Can you work these out from the model? Positions are in its coordinate system, mm. A direction names the side the tool comes from. Coordinates: 2 decimals unless noted, no trailing zeros. Order: outer loops, then holes, each group sorted by start corner. A loop starts at its lowest first (then second) coordinate and runs counter-clockwise, first axis right, second up. Notation, with made-up numbers: (-2, 40.25) -> (50, 40.25) arc R14 ccw to (50, 66.25) -> close; hole circle Ø5 at (16, 69). An arc over 180 degrees is marked (long way). Return JSON: item names as keys, results as strings. Group by question number.
1) If we section it at A-A, the plane x = -13: Please give me the cut outline in (y, z).
2) For pin 1 (5 mm diameter, centred on x = -12.5, y = 6, fed in from +Z); pin 2 (5.5 mm diameter, centred on x = -20, z = 0.5, fed in from +Y); pin 3 (2.5 mm diameter, centred on x = -1.5, z = -0.5, fed in from -Y); pin 4 (5 mm diameter, centred on x = 0.5, y = 3.5, fed in from +Z), each with a flat end and sliding along its axis, tell me the tip position at first contact or that it passes through.
3) If I drill on probe 1 along X at (y, z) = (3.05, 0); probe 2 along Z at (x, y) = (-26, 1.75); probe 3 along Z at (x, y) = (1, 9.75), over which ranges is the centre line in solid material (lowest first)? Write a range as from..to.
4) For faces 1 (the flat face through (-19, 4, 0)), 2 (the flat face through (-3.25, 1.97, -7.81)), 3 (the flat face through (-17, 5, 7)), which set-ups out of +Z, -Z, +X, -X, +Y, -Y let a thin tool reach every point of the face, with its end or its side?
5) If we section it at C-C, the plane y = 7.25: Please give me the cut outline in (x, z), then the cut area to 3 significant figures.
6) If we section it at D-D, the plane z = 10: Please give me the cut outline in (x, y).
7) If we section it at B-B, the plane y = 1.5: Please give me the cut outline in (x, z).
8) Thinking about a two-plate mould opening in Z: for faces 4 (the flat face through (5.643, 4.93, 11.69)), 5 (the flat face through (7.22, 4.93, -6.22)), 6 (the flat face through (3.223, 1.972, -7.929)), 7 (the cylindrical face through (0.1, 2, 17.5)), which applies, +Z half, -Z half, draft (parallel to the pull), parting line (faces both ways), or undercut?
from build123d import *

# Parameters (mm, degrees)
ESQUISSE1_R             = 2
BOSS_EXTRU_1_DEPTH      = 10
ESQUISSE2_W             = 10.2
ESQUISSE2_H             = 6
ENL_V_MAT_EXTRU_1_DEPTH = 20
CHANFREIN1_SIZE         = 2.5
CHANFREIN2_SIZE         = 1.8
ESQUISSE5_R             = 1.6
ENL_V_MAT_EXTRU_4_DEPTH = 7
CHANFREIN4_SIZE         = 2.1
CHANFREIN5_SIZE         = 2
ENL_V_MAT_EXTRU_5_DEPTH = 4
CHANFREIN6_SIZE         = 4
CONG_1_R                = 20


with BuildPart() as part:
    # Esquisse1 → Boss.-Extru.1 (new body)
    with BuildSketch(Plane(origin=(0, 0, 0), x_dir=(1, 0, 0), z_dir=(0, 1, 0))):
        with BuildLine():
            Line((-28, -7), (-7, -7))
            Line((-7, -7), (-4.322606063, -16.251030305))
            ThreePointArc((-4.322606063, -16.251030305), (0, -19.5), (4.322606063, -16.251030305))
            Line((4.322606063, -16.251030305), (7, -7))
            Line((7, -7), (8.983874701, 0))
            Line((8.983874701, 0), (7, 7))
            Line((7, 7), (4.322606063, 16.251030305))
            ThreePointArc((4.322606063, 16.251030305), (0, 19.5), (-4.322606063, 16.251030305))
            Line((-4.322606063, 16.251030305), (-7, 7))
            Line((-7, 7), (-28, 7))
            Line((-28, 7), (-28, -7))
        make_face()
        with Locations(Location((0, 0, 0), (0, 0, 270))):
            Circle(ESQUISSE1_R, mode=Mode.SUBTRACT)
    extrude(amount=BOSS_EXTRU_1_DEPTH)

    # Esquisse2 → Enlèv. mat.-Extru.1 (cut)
    with BuildSketch(Plane.ZY.offset(28)):
        with Locations((0, 7)):
            Rectangle(ESQUISSE2_W, ESQUISSE2_H)
    extrude(amount=-ENL_V_MAT_EXTRU_1_DEPTH, mode=Mode.SUBTRACT)

    # Chanfrein1
    chanfrein1_edges = [part.edges().sort_by_distance(p)[0] for p in [
        (-18, 4, -5.1),
        (-18, 4, 5.1),
    ]]
    chamfer(chanfrein1_edges, length=CHANFREIN1_SIZE)

    # Chanfrein2
    chanfrein2_edges = [part.edges().sort_by_distance(p)[0] for p in [
        (-8, 4, 0),
        (-8, 5.25, -3.85),
        (-8, 5.25, 3.85),
    ]]
    chamfer(chanfrein2_edges, length=CHANFREIN2_SIZE)

    # Esquisse5 → Enlèv. mat.-Extru.4 (cut)
    with BuildSketch(Plane.XZ):
        with Locations(Location((-23, 0, 0), (0, 0, 270))):
            Circle(ESQUISSE5_R)
        with Locations(Location((-13, 0, 0), (0, 0, 270))):
            Circle(ESQUISSE5_R)
    extrude(amount=-ENL_V_MAT_EXTRU_4_DEPTH, mode=Mode.SUBTRACT)

    # Chanfrein4
    chanfrein4_edges = [part.edges().sort_by_distance(p)[0] for p in [
        (-23, 0, 1.6),
        (-13, 0, 1.6),
    ]]
    chamfer(chanfrein4_edges, length=CHANFREIN4_SIZE)

    # Chanfrein5
    chanfrein5_edges = [part.edges().sort_by_distance(p)[0] for p in [
        (-28, 5, -7),
        (-28, 5, 7),
    ]]
    chamfer(chanfrein5_edges, length=CHANFREIN5_SIZE)

    # Esquisse6 → Enlèv. mat.-Extru.5 (cut)
    with BuildSketch(Plane.XZ):
        with BuildLine():
            Line((-3.980786407, -0.391585978), (-2.500022814, -15.44473884))
            ThreePointArc((-2.500022814, -15.44473884), (0.085507989, -17.698094096), (2.487468593, -15.25))
            Line((2.487468593, -15.25), (3.979949748, -0.4))
            ThreePointArc((3.979949748, -0.4), (4, 0), (3.979949748, 0.4))
            Line((3.979949748, 0.4), (2.487468593, 15.25))
            ThreePointArc((2.487468593, 15.25), (0, 17.5), (-2.487468593, 15.25))
            Line((-2.487468593, 15.25), (-3.979949748, 0.4))
            ThreePointArc((-3.979949748, 0.4), (-3.999997766, 0.004227758), (-3.980786407, -0.391585978))
        make_face()
    extrude(amount=-ENL_V_MAT_EXTRU_5_DEPTH, mode=Mode.SUBTRACT)

    # Chanfrein6
    chanfrein6_edges = [part.edges().sort_by_distance(p)[0] for p in [
        (0, 10, -2),
    ]]
    chamfer(chanfrein6_edges, length=CHANFREIN6_SIZE)

    # Congé1
    cong_1_edges = [part.edges().sort_by_distance(p)[0] for p in [
        (8.983874701, 5, 0),
    ]]
    fillet(cong_1_edges, radius=CONG_1_R)


solid = part.part
Result sheet:
{
 "1": {"outline": "(0, -7) -> (10, -7) -> (10, -5.1) -> (6.5, -5.1) -> (4, -2.6) -> (4, -1.6) -> (2.1, -1.6) -> (0, -3.7) -> close; (0, 3.7) -> (2.1, 1.6) -> (4, 1.6) -> (4, 2.6) -> (6.5, 5.1) -> (10, 5.1) -> (10, 7) -> (0, 7) -> close"},
 "2": {"pin 1": "stops at z = 7", "pin 2": "stops at y = 4.65", "pin 3": "stops at y = 4", "pin 4": "stops at z = 19.5"},
 "3": {"probe 1": "x = -28..-24.6, -21.4..-14.6, -11.4..-4, 4..8.2", "probe 2": "z = -7..7", "probe 3": "z = -19.39..-5.66, 5.66..19.39"},
 "4": {"face 1": "-X, +Y", "face 2": "-Y", "face 3": "+Z, -X, +Y, -Y"},
 "5": {"outline": "(-27.9, -5.1) -> (-26, -7) -> (-7, -7) -> (-4.32, -16.25) arc R4.5 ccw to (4.32, -16.25) -> (7, -7) -> (7.44, -5.45) arc R20 ccw to (7.44, 5.45) -> (7, 7) -> (4.32, 16.25) arc R4.5 ccw to (-4.32, 16.25) -> (-7, 7) -> (-26, 7) -> (-27.9, 5.1) -> (-9.27, 5.1) -> (-8, 3.3) -> (-8, -3.3) -> (-9.27, -5.1) -> close; hole circle Ø6.5 at (0, 0)", "area": "513 mm2"},
 "6": {"outline": "(-6.13, 0) -> (-3.02, 0) -> (-3.02, 4) -> (3.02, 4) -> (3.02, 0) -> (6.13, 0) -> (6.13, 10) -> (-6.13, 10) -> close"},
 "7": {"outline": "(-28, -5) -> (-26, -7) -> (-7, -7) -> (-4.32, -16.25) arc R4.5 ccw to (4.32, -16.25) -> (7, -7) -> (7.44, -5.45) arc R20 ccw to (7.44, 5.45) -> (7, 7) -> (4.32, 16.25) arc R4.5 ccw to (-4.32, 16.25) -> (-7, 7) -> (-26, 7) -> (-28, 5) -> close; hole circle Ø4.4 at (-23, 0); hole circle Ø4.4 at (-13, 0); hole (-3.98, -0.39) -> (-2.5, -15.44) arc R2.5 ccw to (2.49, -15.25) -> (3.98, -0.4) arc R4 ccw to (3.98, 0.4) -> (2.49, 15.25) arc R2.5 ccw to (-2.49, 15.25) -> (-3.98, 0.4) arc R4 ccw to start"},
 "8": {"face 4": "+Z half", "face 5": "-Z half", "face 6": "undercut", "face 7": "undercut"}
}
